The listing builds one solid part. Answer for the finished solid, in the listing's coordinates (mm). A direction names the side the tool comes from. Coordinates: 2 decimals unless noted, no trailing zeros. Order: outer loops, then holes, each group sorted by start corner. A loop starts at its lowest first (then second) coordinate and runs counter-clockwise, first axis right, second up. Notation, with made-up numbers: (21, -12.75) -> (56, -12.75) arc R18 ccw to (56, 4.25) -> close; hole circle Ø10 at (20, 58). An arc over 180 degrees is marked (long way). Answer in a Markdown table with one row per item.
Autodesk Inventor part; units mm, degrees
ref_plane "YZ Plane" through (0, 0, 0) normal (1, 0, 0) x (0, 1, 0)
ref_plane "XZ Plane" through (0, 0, 0) normal (0, 1, 0) x (-1, 0, 0)
ref_plane "XY Plane" through (0, 0, 0) normal (0, 0, 1) x (1, 0, 0)
sketch "Sketch1" plane through (0, 0, 0) normal (1, 0, 0) x (0, 1, 0)
  line L0 (0, 0) -> (107.95, 0)
  line L1 (107.95, 0) -> (107.95, -57.15)
  line L2 (107.95, -57.15) -> (0, -57.15)
  line L3 (0, -57.15) -> (0, 0)
  line L4 (107.95, -57.15) -> (25.4, -57.15)
  line L5 (25.4, -57.15) -> (25.4, -25.4)
  line L6 (25.4, -25.4) -> (107.95, -25.4)
  line L7 (107.95, -25.4) -> (107.95, -57.15)
  dimension "d0" = 107.95
  dimension "d1" = 57.15
  dimension "d2" = 82.55
  dimension "d3" = 31.75
extrude "Extrusion1" add sketch "Sketch1" along normal blind 6.35 contours L0 L1 L6 L5 L2 L3
sketch "Sketch2" plane through (6.35, 0, 0) normal (1, 0, 0) x (0, 0, -1)
  line L0 (0, 0) -> (57.15, 0)
  line L1 (57.15, 25.4) -> (25.4, 25.4)
  line L2 (25.4, 25.4) -> (25.4, 107.95)
  line L3 (25.4, 107.95) -> (0, 107.95)
  line L4 (0, 107.95) -> (0, 0)
  line L5 (0, 0) -> (57.15, 0)
  line L6 (57.15, 0) -> (57.15, 25.4)
  point P0 (4.699, 92.9894)
  point P1 (20.701, 92.9894)
  dimension "d6" = 92.9894
  dimension "d7" = 92.9894
  dimension "d8" = 16.002
  dimension "d9" = 25.4
  dimension "d10" = 4.699
hole "Hole1" at (6.35, 92.9894, -4.699) at (6.35, 92.9894, -20.701) direction (-1, 0, 0) diameter 3.81 end through all
sketch "Sketch3" plane through (6.35, 0, 0) normal (1, 0, 0) x (0, 0, -1)
  line L0 (57.15, 25.4) -> (25.4, 25.4)
  line L1 (57.15, 0) -> (57.15, 25.4)
  point P0 (0, 0)
  point P1 (44.45, 12.7)
  dimension "d18" = 12.7
  dimension "d19" = 12.7
hole "Hole2" at (6.35, 12.7, -44.45) direction (-1, 0, 0) diameter 8.128 end through all
sketch "Sketch4" plane through (6.35, 0, 0) normal (1, 0, 0) x (0, 0, -1)
  line L0 (0, 107.95) -> (0, 0)
  line L1 (0, 0) -> (57.15, 0)
  line L2 (25.4, 25.4) -> (25.4, 107.95)
  point P0 (12.1412, 76.2)
  point P1 (12.1412, 38.1)
  dimension "d29" = 38.1
  dimension "d30" = 76.2
  dimension "d38" = 13.2588
  dimension "d39" = 13.2588
hole "Hole3" at (6.35, 76.2, -12.1412) at (6.35, 38.1, -12.1412) direction (-1, 0, 0) diameter 3.81 depth 10.9728 tip angle 118
sketch "Sketch5" plane through (0, 0, 0) normal (0, 0, 1) x (1, 0, 0)
  line L0 (0, 107.95) -> (0, 0)
  line L1 (0, 0) -> (6.35, 0)
  line L2 (6.35, 107.95) -> (6.35, 0)
  line L3 (0, 107.95) -> (6.35, 107.95)
extrude "Extrusion2" add sketch "Sketch5" along normal blind 6.35
sketch "Sketch6" plane through (6.35, 0, 0) normal (1, 0, 0) x (0, 0, -1)
  line L0 (-6.35, 0) -> (-6.35, 107.95)
  line L1 (57.15, 0) -> (-6.35, 0)
  point P0 (0, 0)
  point P1 (-1.5875, 17.4625)
  point P2 (-1.5875, 7.9375)
  dimension "d42" = 4.7625
  dimension "d43" = 4.7625
  dimension "d44" = 9.525
  dimension "d45" = 7.9375
hole "Hole4" at (6.35, 17.4625, 1.5875) at (6.35, 7.9375, 1.5875) direction (-1, 0, 0) diameter 3.81 end through all
properties part number "PaddleCollection2.1ServoSupport" material "Nylon 6/6"
(1) Find the intervals of material crossed by line 1 along Y through (x, z) = (2.5, -44.45); line 2 along Y through (x, z) = (3.75, -44); line 3 along Z through (x, y) = (3, 12.7), in increasing order. Write a range as from..to.
Check values:
| item | result |
|---|---|
| line 1 | 0..8.64, 16.76..25.4 |
| line 2 | 0..8.66, 16.74..25.4 |
| line 3 | -57.15..-48.51, -40.39..6.35 |
(2) Which of the six approach directions +Z, -Z, +X, -X, +Y, -Y give full straight-line access (tool end or side, diameter ignored) to faces 1 (the flat face through (3, 66, -25.4)), 2 (the cylindrical face through (3.131, 6.331, 0.563))?
Check values:
| item | result |
|---|---|
| face 1 | -Z, +X, -X, +Y |
| face 2 | +X, -X |
(3) A cutting plane is placed at B-B, the plane y = 12.7. Determine the outline of the cut face in (x, z).
Check values:
| item | result |
|---|---|
| outline | (0, -57.15) -> (6.35, -57.15) -> (6.35, -48.51) -> (0, -48.51) -> close; (0, -40.39) -> (6.35, -40.39) -> (6.35, 6.35) -> (0, 6.35) -> close |
(4) For a pull along Z with two mould halves and no side action, classify faces 3 (the flat face through (3, 55, 6.35)), 4 (the flat face through (3, 0, -26)), 5 (the cylindrical face through (3.13, 74.31, -11.89)) as released by +Z, released by -Z, zero draft, split by the parting line, or undercut.
Check values:
| item | result |
|---|---|
| face 3 | released by +Z |
| face 4 | zero draft |
| face 5 | undercut |
(5) Flat-ended cylindrical pins translate along their axes: pin 1 (3.5 mm diameter, centred on y = 76.2, z = -12.14, fed in from +X); pin 2 (6 mm diameter, centred on y = 92.99, z = -20.7, fed in from +X). Find the tip coordinate at first contact, or state that the pin passes through.
Check values:
| item | result |
|---|---|
| pin 1 | through |
| pin 2 | x = 6.35 |
(6) A cutting plane is placed at C-C, the plane x = 1.5. Count the separate pieces of the cut face and the enclosed holes in it, then the cut area to 3 significant figures.
Check values:
| item | result |
|---|---|
| separate pieces | 1 |
| enclosed holes | 7 |
| area | 4,110 mm² |
(7) A cutting plane is placed at A-A, the plane z = -44.45. Determine the outline of the cut face in (x, y).
Check values:
| item | result |
|---|---|
| outline | (0, 0) -> (6.35, 0) -> (6.35, 8.64) -> (0, 8.64) -> close; (0, 16.76) -> (6.35, 16.76) -> (6.35, 25.4) -> (0, 25.4) -> close |
